Model file for the job. Use its own axes, mm. A direction names the side the tool comes from. Give positions to 0.01 mm unless a question says otherwise; leave off trailing zeros. Order: outer loops, then holes, each group sorted by start corner. A loop starts at its lowest first (then second) coordinate and runs counter-clockwise, first axis right, second up. Notation, with made-up numbers: (84, 65.25) - (90, 65.25) arc R14 cw to (90, 83.25) - close; hole circle Ø3 at (-6.75, 37). An arc over 180 degrees is marked (long way). Return JSON: item names as keys, results as strings. Group by question number.
from build123d import *

# Parameters (mm, degrees)
SKETCH1_W           = 6.1
SKETCH1_H           = 3.55
BOSS_EXTRUDE1_DEPTH = 3.21
SKETCH2_W           = 2.95
SKETCH2_H           = 1.45
BOSS_EXTRUDE2_DEPTH = 1
BOSS_EXTRUDE3_DEPTH = 0.2
EXTRUDE_THIN1_DEPTH = 0.5


with BuildPart() as part:
    # Sketch1 → Boss-Extrude1 (new body)
    with BuildSketch(Plane(origin=(0, 0, 0), x_dir=(1, 0, 0), z_dir=(0, 1, 0))):
        Rectangle(SKETCH1_W, SKETCH1_H)
    extrude(amount=BOSS_EXTRUDE1_DEPTH)

    # Sketch2 → Boss-Extrude2 (add)
    with BuildSketch(Plane(origin=(0, 3.21, 0), x_dir=(1, 0, 0), z_dir=(0, 1, 0))):
        Rectangle(SKETCH2_W, SKETCH2_H)
    extrude(amount=BOSS_EXTRUDE2_DEPTH)

    # Sketch3 → Boss-Extrude3 (add)
    with BuildSketch(Plane(origin=(0, 3.21, 0), x_dir=(1, 0, 0), z_dir=(0, 1, 0))):
        with BuildLine():
            Line((-2.0125, 0.85), (-2.0125, -0.85))
            ThreePointArc((-2.0125, -0.85), (-2.2625, -1.1), (-2.5125, -0.85))
            Line((-2.5125, -0.85), (-2.5125, 0.85))
            ThreePointArc((-2.5125, 0.85), (-2.2625, 1.1), (-2.0125, 0.85))
        make_face()
        with BuildLine():
            Line((2.0125, 0.85), (2.0125, -0.85))
            ThreePointArc((2.0125, -0.85), (2.2625, -1.1), (2.5125, -0.85))
            Line((2.5125, -0.85), (2.5125, 0.85))
            ThreePointArc((2.5125, 0.85), (2.2625, 1.1), (2.0125, 0.85))
        make_face()
    extrude(amount=BOSS_EXTRUDE3_DEPTH)

    # Sketch4 → Extrude-Thin1 (add, symmetric)
    with BuildSketch(Plane.XY):
        Polygon((-2.653608324, 1.60852371), (-3.96, 0.302132034), (-3.96, -3), (-3.66, -3), (-3.66, 0.177867966), (-2.44147629, 1.396391676), align=None)
        Polygon((2.44147629, 1.396391676), (3.66, 0.177867966), (3.66, -3), (3.96, -3), (3.96, 0.302132034), (2.653608324, 1.60852371), align=None)
    extrude(amount=EXTRUDE_THIN1_DEPTH, both=True)


solid = part.part
(1) Slice it at B-B (x = -0.25). Give the cut face in (y, z) (3 decimals), and give its area (3 significant figures).
(2) Drop flat-ended pins along their axis: pin 1 Ø0.5 at (x, y) = (-0.5, 4) entering from -Z (3 decimals); pin 2 Ø1 at (x, y) = (-3.5, -1) entering from +Z; pin 3 Ø1.1 at (y, z) = (3.5, 0.5) entering from +X; pin 4 Ø2 at (x, y) = (-0.5, -1.5) entering from +Z. Give the stop position or say it passes through.
(3) Pull direction X, two halves, no side cores. Call faces 1 (the face through (-3.96, -1, 0)), 2 (the face through (0, 3.21, 1)), 3 (the face through (0, 4.21, 0)): released by +X, released by -X, zero draft, split by the parting line, or undercut.
(4) Slice it at A-A (y = -2.5). Give the cut face in (x, z), and give its area (3 significant figures).
(5) Drill centre lines: L1, parallel to X at y = -2.5, z = -0.4; L2, parallel to Y at x = -1.25, z = -0.2; L3, parallel to Y at x = -1.75, z = 1.05. Where is each one in solid material? Low to high.
(6) 3-axis set-ups, long thin cutter, end or side, ignore diameter. For faces 4 (the face through (3.66, -1, 0)), 5 (the face through (0, 4, 0.725)), 6 (the face through (-1.475, 4, 0)): which of +Z, -Z, +X, -X, +Y, -Y reach the whole face in a straight line?
(7) Slice it at D-D (y = 0.5). Give the cut face in (x, z) (3 decimals).
Result set:
{
 "1": {"outline": "(0, -1.775) - (3.21, -1.775) - (3.21, -0.725) - (4.21, -0.725) - (4.21, 0.725) - (3.21, 0.725) - (3.21, 1.775) - (0, 1.775) - close", "area": "12.8 mm²"},
 "2": {"pin 1": "stops at z = -0.725", "pin 2": "stops at z = 0.5", "pin 3": "stops at x = 3.05", "pin 4": "passes through"},
 "3": {"face 1": "released by -X", "face 2": "undercut", "face 3": "zero draft"},
 "4": {"outline": "(-3.96, -0.5) - (-3.66, -0.5) - (-3.66, 0.5) - (-3.96, 0.5) - close; (3.66, -0.5) - (3.96, -0.5) - (3.96, 0.5) - (3.66, 0.5) - close", "area": "0.600 mm²"},
 "5": {"L1": "x = -3.96 to -3.66, 3.66 to 3.96", "L2": "y = 0 to 4.21", "L3": "y = 0 to 3.21"},
 "6": {"face 4": "+Z, -Z, -Y", "face 5": "+Z, +Y", "face 6": "+Z, -Z, +Y"},
 "7": {"outline": "(-3.762, -0.5) - (-3.338, -0.5) - (-3.338, 0.5) - (-3.762, 0.5) - close; (-3.05, -1.775) - (3.05, -1.775) - (3.05, 1.775) - (-3.05, 1.775) - close; (3.338, -0.5) - (3.762, -0.5) - (3.762, 0.5) - (3.338, 0.5) - close"}
}
